Model file for the job. Use its own axes, mm. A direction names the side the tool comes from. Round coordinates to 2 decimals unless told otherwise and drop trailing zeros. Write each loop counter-clockwise with the first axis right and the second up, starting at its lowest first coordinate (ties: lowest second). Pieces come first, ordered by that corner, then holes.
Autodesk Inventor part; units mm, degrees
ref_plane "YZ Plane" through (0, 0, 0) normal (1, 0, 0) x (0, 1, 0)
ref_plane "XZ Plane" through (0, 0, 0) normal (0, 1, 0) x (-1, 0, 0)
ref_plane "XY Plane" through (0, 0, 0) normal (0, 0, 1) x (1, 0, 0)
sketch "Sketch1" plane through (0, 0, 0) normal (0, 1, 0) x (-1, 0, 0)
  line L0 (5.3, -5.3) -> (-5.3, -5.3)
  line L1 (-5.3, -5.3) -> (-5.3, 5.3)
  line L2 (-5.3, 5.3) -> (5.3, 5.3)
  line L3 (5.3, 5.3) -> (5.3, -5.3)
  line L4 (7.8, -5.3) -> (7.8, 5.3)
  line L5 (-7.8, 5.3) -> (-7.8, -5.3)
  line L6 (5.3, -5.3) -> (7.8, -5.3)
  line L7 (-5.3, -5.3) -> (-7.8, -5.3)
  line L8 (-5.3, 5.3) -> (-7.8, 5.3)
  line L9 (5.3, 5.3) -> (7.8, 5.3)
  point P0 (0, 0)
  point P1 (-5.3, 0)
  point P2 (0, -5.3)
  dimension "d0" = 10.6
  dimension "d1" = 10.6
extrude "Extrusion1" add sketch "Sketch1" along normal blind 2
extrude "Extrusion2" add sketch "Sketch1" along normal blind 5 contours L3 L9 L4 L6 | L7 L5 L8 L1
sketch "Sketch2" plane through (-5.3, 2, -5.3) normal (1, 0, 0) x (0, 0, -1)
  line L0 (0, 0) -> (-10.6, 0)
  line L1 (0, 0) -> (0, 3)
  line L2 (-10.6, 3) -> (0, 3)
  line L3 (-10.6, 0) -> (-10.6, 3)
  line L4 (-10.6, 3) -> (0, 3)
  line L5 (0, 3) -> (0, 2)
  line L6 (0, 2) -> (-10.6, 2)
  line L7 (-10.6, 2) -> (-10.6, 3)
  point P0 (-5.3, -2)
  dimension "d7" = 1
extrude "Extrusion3" add sketch "Sketch2" along normal blind 2 contours L6 L3 L2 L1
mirror "Mirror1" about plane through (0, 0, 0) normal (1, 0, 0) of "Extrusion3"
move faces "Move1" translate (0, -2, 0) faces at (-2.6, 0, 1.7667)
sketch "Sketch3" plane through (-7.8, -2, -5.3) normal (0, -1, 0) x (1, 0, 0)
  line L0 (15.6, 0) -> (0, 0)
  line L1 (15.6, 10.6) -> (15.6, 0)
  line L2 (0, 10.6) -> (15.6, 10.6)
  line L3 (0, 0) -> (0, 10.6)
  line L4 (7.8, 10.6) -> (7.8, 0)
  circle A0 centre (7.8, 5.3) radius 2
  dimension "d13" = 4
extrude "Extrusion4" cut sketch "Sketch3" against normal through all contours A0 L4 | L4 A0
sketch "Sketch4" plane through (0, 2, 0) normal (0, 1, 0) x (1, 0, 0)
  circle A0 centre (0, 0) radius 2
  line L0 (-5.3, 5.3) -> (-5.3, -5.3)
  line L1 (-5.3, -5.3) -> (5.3, -5.3)
  line L2 (5.3, -5.3) -> (5.3, 5.3)
  line L3 (5.3, 5.3) -> (-5.3, 5.3)
  circle A1 centre (0, 0) radius 4
  dimension "d16" = 2
extrude "Extrusion5" cut sketch "Sketch4" against normal blind 2 contours A1
properties part number "MicroUSBClip"
1) Cut at B-B on z = 0. List the corners of the cut face in (x, y).
2) Cut at A-A on y = 3.25. List the corners of the cut face in (x, z).
3) Flat gauge pin, fed straight in: pin 1 Ø5 at (x, z) = (0, 0) entering from -Y. Where does the tip first touch, or does it go through?
4) Wall check: probe 1 along X at (y, z) = (-0.5, 0); probe 2 along Y at (x, z) = (-4, 0.5); probe 3 along Z at (x, y) = (0, -0.55). Give the ranges that are in metal, low to high.
5) Cut at D-D on y = -0.75. List the corners of the cut face in (x, z), and give its area (3 significant figures).
6) Pull direction X, two halves, no side cores. Call faces 1 (the face through (7.8, 1, 0)), 2 (the face through (-5.3, 3, 0)), 3 (the face through (0, 1, -5.3)): released by +X, released by -X, zero draft, split by the parting line, or undercut.
7) Cut at C-C on x = 0. List the corners of the cut face in (y, z), and give its area (3 significant figures).
8) Which spindle directions (+Z, -Z, +X, -X, +Y, -Y) get a long thin tool onto all of the face, cutting with end or side? Do faces 4 (the face through (-0.867, 1.014, 3.905)), 5 (the face through (3.3, 4.5, -0.1)), 6 (the face through (-6, 5, 0)), 7 (the face through (-4, 4, 0)). Say none if no direction does.
Result sheet:
1. outline: (-7.8, -2) - (-2, -2) - (-2, 0) - (-4, 0) - (-4, 2) - (-5.3, 2) - (-5.3, 4) - (-3.3, 4) - (-3.3, 5) - (-7.8, 5) - close; (2, -2) - (7.8, -2) - (7.8, 5) - (3.3, 5) - (3.3, 4) - (5.3, 4) - (5.3, 2) - (4, 2) - (4, 0) - (2, 0) - close
2. outline: (-7.8, -5.3) - (-5.3, -5.3) - (-5.3, 5.3) - (-7.8, 5.3) - close; (5.3, -5.3) - (7.8, -5.3) - (7.8, 5.3) - (5.3, 5.3) - close
3. pin 1: stops at y = -2
4. probe 1: x = -7.8 to -2, 2 to 7.8
4. probe 2: y = -2 to 2, 4 to 5
4. probe 3: z = -5.3 to -2, 2 to 5.3
5. outline: (-7.8, -5.3) - (7.8, -5.3) - (7.8, 5.3) - (-7.8, 5.3) - close; hole circle Ø4 at (0, 0)
5. area: 153 mm2
6. face 1: released by +X
6. face 2: undercut
6. face 3: zero draft
7. outline: (-2, -5.3) - (2, -5.3) - (2, -4) - (0, -4) - (0, -2) - (-2, -2) - close; (-2, 2) - (0, 2) - (0, 4) - (2, 4) - (2, 5.3) - (-2, 5.3) - close
7. area: 18.4 mm2
8. face 4: none
8. face 5: +Z, -Z, +Y
8. face 6: +Z, -Z, +X, -X, +Y
8. face 7: +Z, -Z
